from build123d import *

# Parameters (mm, degrees)
EXTRUDE_START       = -7.5
EXTRUDE_1_DEPTH     = 15
SKETCH_2_R          = 5.5
CUT_EXTRUDE_1_DEPTH = 6
SKETCH_3_R          = 3.3
CUT_EXTRUDE_2_DEPTH = 123.805740908


# Read off the part's stored shape, not the designer's step: 凸台-拉伸1
with BuildPart() as part:
    # 凸台-拉伸1 outline → 凸台-拉伸1 (new body)
    with BuildSketch(Plane.XY.offset(EXTRUDE_START)):
        Polygon((0, 0), (120, 0), (120, 20), (118.319851, 20), (116.5, 25), (113.5, 25), (111.680149, 20), (108.319851, 20), (106.5, 25), (103.5, 25), (101.680149, 20), (98.319851, 20), (96.5, 25), (93.5, 25), (91.680149, 20), (88.319851, 20), (86.5, 25), (83.5, 25), (81.680149, 20), (78.319851, 20), (76.5, 25), (73.5, 25), (71.680149, 20), (68.319851, 20), (66.5, 25), (63.5, 25), (61.680149, 20), (58.319851, 20), (56.5, 25), (53.5, 25), (51.680149, 20), (48.319851, 20), (46.5, 25), (43.5, 25), (41.680149, 20), (38.319851, 20), (36.5, 25), (33.5, 25), (31.680149, 20), (28.319851, 20), (26.5, 25), (23.5, 25), (21.680149, 20), (18.319851, 20), (16.5, 25), (13.5, 25), (11.680149, 20), (8.319851, 20), (6.5, 25), (3.5, 25), (1.680149, 20), (0, 20), align=None)
    extrude(amount=EXTRUDE_1_DEPTH)

    # 草图2 → 切除-拉伸1 (cut)
    with BuildSketch(Plane(origin=(0, 0, 0), x_dir=(1, 0, 0), z_dir=(0, 1, 0))):
        with Locations(Location((30, 0, 0), (0, 0, 270))):
            Circle(SKETCH_2_R)
        with Locations(Location((90, 0, 0), (0, 0, 270))):
            Circle(SKETCH_2_R)
    extrude(amount=CUT_EXTRUDE_1_DEPTH, mode=Mode.SUBTRACT)

    # 草图3 → 切除-拉伸2 (cut, through all)
    with BuildSketch(Plane(origin=(0, 0, 0), x_dir=(1, 0, 0), z_dir=(0, 1, 0))):
        with Locations(Location((30, 0, 0), (0, 0, 120.606300293))):
            Circle(SKETCH_3_R)
        with Locations(Location((90, 0, 0), (0, 0, 120.606300293))):
            Circle(SKETCH_3_R)
    extrude(amount=CUT_EXTRUDE_2_DEPTH, mode=Mode.SUBTRACT)


solid = part.part
Check sheet for the modelled part. Datum: model origin and axes. Units: mm. A direction names the side the tool comes from. Give positions to 0.01 mm unless a question says otherwise; leave off trailing zeros. Write each loop counter-clockwise with the first axis right and the second up, starting at its lowest first coordinate (ties: lowest second). Pieces come first, ordered by that corner, then holes. Notation, with made-up numbers: (64.25, 33) -> (101.25, 33) arc R13 ccw to (101.25, 40) -> close; hole circle Ø5 at (30, -2). An arc over 180 degrees is marked (long way). Write item = value, one per line.
Item 1: Sectioned sample at A-A on x = 90. Record the boundary of the cut face in (y, z).
Output:
outline = (0, -7.5) -> (20, -7.5) -> (20, -3.3) -> (6, -3.3) -> (6, -5.5) -> (0, -5.5) -> close; (0, 5.5) -> (6, 5.5) -> (6, 3.3) -> (20, 3.3) -> (20, 7.5) -> (0, 7.5) -> close
Item 2: Sectioned sample at C-C on z = 0. Count the separate pieces of the cut face and the enclosed holes in it, and give its area (3 significant figures).
Output:
separate_pieces = 3
enclosed_holes = 0
area = 2,360 mm^2
Item 3: Sectioned sample at D-D on y = 2. Record the boundary of the cut face in (x, z), and give its area (3 significant figures).
Output:
outline = (0, -7.5) -> (120, -7.5) -> (120, 7.5) -> (0, 7.5) -> close; hole circle Ø11 at (30, 0); hole circle Ø11 at (90, 0)
area = 1,610 mm^2
Item 4: Scan lines: probe 1 along X at (y, z) = (4, -0.5); probe 2 along X at (y, z) = (17.75, 0); probe 3 along Z at (x, y) = (30, 14). Record each from-to range of solid material in increasing order. Write a range as from..to.
Output:
probe_1 = 0..24.52, 35.48..84.52, 95.48..120
probe_2 = 0..26.7, 33.3..86.7, 93.3..120
probe_3 = -7.5..-3.3, 3.3..7.5
Item 5: Gauge pin test, flat end, axial feed: pin 1 (1.3 mm diameter, centred on x = 0.5, z = 1, fed in from +Y). Record the tip position at first contact, or that the pin passes through.
Output:
pin_1 = 20
Item 6: Tool access check on faces 1 (the flat face through (75, 25, 0)), 2 (the cylindrical face through (95.453, 2.958, -0.716)), 3 (the flat face through (50, 20, 0)). Record the directions out of +Z, -Z, +X, -X, +Y, -Y that give a thin tool (end or side, any length) a straight path to the whole face; none if there is none.
Output:
face_1 = +Z, -Z, +X, -X, +Y
face_2 = -Y
face_3 = +Z, -Z, +Y
Item 7: Release check for a two-part mould opening along X. For faces 4 (the flat face through (15, 25, 0)), 5 (the flat face through (72.603, 22.535, -0.105)) record: +X half, -X half, draft (parallel to the pull), parting line (faces both ways), or undercut.
Output:
face_4 = draft
face_5 = undercut
Item 8: Sectioned sample at B-B on y = 15.5. Record the boundary of the cut face in (x, z), and give its area (3 significant figures).
Output:
outline = (0, -7.5) -> (120, -7.5) -> (120, 7.5) -> (0, 7.5) -> close; hole circle Ø6.6 at (30, 0); hole circle Ø6.6 at (90, 0)
area = 1,730 mm^2
